Design review of the part built by this model. Coordinates are the model's own, in mm. A direction names the side the tool comes from. Round coordinates to 2 decimals unless told otherwise and drop trailing zeros. Order: outer loops, then holes, each group sorted by start corner. A loop starts at its lowest first (then second) coordinate and runs counter-clockwise, first axis right, second up. Notation, with made-up numbers: (88.25, -26.5) - (136.25, -26.5) arc R32 cw to (136.25, 8.5) - close; hole circle Ø5 at (23, 71). An arc over 180 degrees is marked (long way). Write item = value, one per line.
from build123d import *

# Parameters (mm, degrees)
CYLINDER2172_R               = 56
CYLINDER2172_DEPTH           = 7
CYLINDER2171_R               = 51
CYLINDER2171_DEPTH           = 7
BOX1045_W                    = 1.4
BOX1045_H                    = 60
BOX1045_DEPTH                = 7
BOX1045_PLACEMENT_ANGLE      = 19.7
BOX1044_W                    = 1.4
BOX1044_H                    = 60
BOX1044_DEPTH                = 7
BOX1044_PLACEMENT_ANGLE      = 18
CUT727_PLACEMENT_ANGLE       = 45
BOX1038_W                    = 60
BOX1038_H                    = 60
BOX1038_DEPTH                = 7
BOX1038_PLACEMENT_ANGLE      = 1
BOX1036_W                    = 60
BOX1036_H                    = 60
BOX1036_DEPTH                = 7
BOX1036_PLACEMENT_ANGLE      = 2
BOX1043_W                    = 120
BOX1043_H                    = 60
BOX1043_DEPTH                = 7
TUBE090_R                    = 54.4
TUBE090_R_2                  = 53
TUBE090_DEPTH                = 7
BOX1041_W                    = 60
BOX1041_H                    = 60
BOX1041_DEPTH                = 7
BOX1041_PLACEMENT_ANGLE      = 20
BOX1039_W                    = 60
BOX1039_H                    = 60
BOX1039_DEPTH                = 7
BOX1039_PLACEMENT_ANGLE      = 20
BOX1037_W                    = 120
BOX1037_H                    = 60
BOX1037_DEPTH                = 7
TUBE091_R                    = 53.4
TUBE091_R_2                  = 52
TUBE091_DEPTH                = 7
CUT721_PLACEMENT_ANGLE       = 45
CYLINDER2170_R               = 51
CYLINDER2170_DEPTH           = 7
BOX1042_W                    = 1.4
BOX1042_H                    = 60
BOX1042_DEPTH                = 7
BOX1042_PLACEMENT_ANGLE      = 2.7
BOX1040_W                    = 1.4
BOX1040_H                    = 60
BOX1040_DEPTH                = 7
BOX1040_PLACEMENT_ANGLE      = 2
CUT722_PLACEMENT_ANGLE       = 45
CYLINDER2129_R               = 1.5
CYLINDER2129_DEPTH           = 100
CYLINDER2130_R               = 1.5
CYLINDER2130_DEPTH           = 100
CYLINDER2130_PLACEMENT_ANGLE = 145
CYLINDER2131_R               = 1.5
CYLINDER2131_DEPTH           = 100
CYLINDER2132_R               = 1.5
CYLINDER2132_DEPTH           = 100
CYLINDER2132_PLACEMENT_ANGLE = 225
CYLINDER2133_R               = 1.5
CYLINDER2133_DEPTH           = 100
CYLINDER2134_R               = 1.5
CYLINDER2134_DEPTH           = 100
CYLINDER2134_PLACEMENT_ANGLE = 45
CYLINDER2127_R               = 1.5
CYLINDER2127_DEPTH           = 100
CYLINDER2128_R               = 1.5
CYLINDER2128_DEPTH           = 100
CYLINDER2128_PLACEMENT_ANGLE = 45
TUBE092_R                    = 57
TUBE092_R_2                  = 32
TUBE092_DEPTH                = 10


with BuildPart() as obj1:
    # Cylinder2172 → Cylinder2172 (new body)
    with BuildSketch(Plane.XY.offset(45)):
        Circle(CYLINDER2172_R)
    extrude(amount=CYLINDER2172_DEPTH)


with BuildPart() as obj2:
    # Cylinder2171 → Cylinder2171 (new body)
    with BuildSketch(Plane.XY.offset(-22)):
        Circle(CYLINDER2171_R)
    extrude(amount=CYLINDER2171_DEPTH)


with BuildPart() as krychle1045:
    # Box1045 → Box1045 (new body)
    with BuildSketch(Plane.XY):
        with Locations((0.7, 30)):
            Rectangle(BOX1045_W, BOX1045_H)
    extrude(amount=BOX1045_DEPTH)


with BuildPart() as krychle1045_1:
    # Box1045 placement: moved
    add(krychle1045.part.moved(Location((0, 0, -22))).rotate(Axis((0, 0, -22), (0, 0, 1)), BOX1045_PLACEMENT_ANGLE))


with BuildPart() as common:
    # Box1044 → Box1044 (new body)
    with BuildSketch(Plane.XY):
        with Locations((0.7, 30)):
            Rectangle(BOX1044_W, BOX1044_H)
    extrude(amount=BOX1044_DEPTH)


with BuildPart() as common_1:
    # Box1044 placement: moved
    add(common.part.moved(Location((0, 0, -22))).rotate(Axis((0, 0, -22), (0, 0, -1)), BOX1044_PLACEMENT_ANGLE))

    # Compound1133: union Krychle1045
    add(krychle1045_1.part)

    # Cut727: cut obj2
    add(obj2.part, mode=Mode.SUBTRACT)


with BuildPart() as common_2:
    # Cut727 placement: moved
    add(common_1.part.moved(Location((0, 0, 67))).rotate(Axis((0, 0, 67), (0, 0, 1)), CUT727_PLACEMENT_ANGLE))

    # Common: intersect obj1
    add(obj1.part, mode=Mode.INTERSECT)


with BuildPart() as krychle1038:
    # Box1038 → Box1038 (new body)
    with BuildSketch(Plane.XY):
        with Locations((30, 30)):
            Rectangle(BOX1038_W, BOX1038_H)
    extrude(amount=BOX1038_DEPTH)


with BuildPart() as krychle1038_1:
    # Box1038 placement: moved
    add(krychle1038.part.moved(Location((-59.990862, -1.047144, -22))).rotate(Axis((-59.990862, -1.047144, -22), (0, 0, 1)), BOX1038_PLACEMENT_ANGLE))


with BuildPart() as compound1130:
    # Box1036 → Box1036 (new body)
    with BuildSketch(Plane.XY):
        with Locations((30, 30)):
            Rectangle(BOX1036_W, BOX1036_H)
    extrude(amount=BOX1036_DEPTH)


with BuildPart() as compound1130_1:
    # Box1036 placement: moved
    add(compound1130.part.moved(Location((0, 0, -22))).rotate(Axis((0, 0, -22), (0, 0, -1)), BOX1036_PLACEMENT_ANGLE))

    # Compound1130: union Krychle1038
    add(krychle1038_1.part)


with BuildPart() as krychle1043:
    # Box1043 → Box1043 (new body)
    with BuildSketch(Plane(origin=(-60, -60, -22), x_dir=(1, 0, 0), z_dir=(0, 0, 1))):
        with Locations((60, 30)):
            Rectangle(BOX1043_W, BOX1043_H)
    extrude(amount=BOX1043_DEPTH)


with BuildPart() as cut723:
    # Tube090 → Tube090 (new body)
    with BuildSketch(Plane.XY.offset(-22)):
        Circle(TUBE090_R)
        Circle(TUBE090_R_2, mode=Mode.SUBTRACT)
    extrude(amount=TUBE090_DEPTH)

    # Cut726: cut Krychle1043
    add(krychle1043.part, mode=Mode.SUBTRACT)

    # Cut723: cut Compound1130
    add(compound1130_1.part, mode=Mode.SUBTRACT)


with BuildPart() as cut723_1:
    # Cut723 placement: moved
    add(cut723.part.moved(Location((0, 0, -7))))


with BuildPart() as krychle1041:
    # Box1041 → Box1041 (new body)
    with BuildSketch(Plane.XY):
        with Locations((30, 30)):
            Rectangle(BOX1041_W, BOX1041_H)
    extrude(amount=BOX1041_DEPTH)


with BuildPart() as krychle1041_1:
    # Box1041 placement: moved
    add(krychle1041.part.moved(Location((-56.381557, -20.521209, -22))).rotate(Axis((-56.381557, -20.521209, -22), (0, 0, 1)), BOX1041_PLACEMENT_ANGLE))


with BuildPart() as compound1129:
    # Box1039 → Box1039 (new body)
    with BuildSketch(Plane.XY):
        with Locations((30, 30)):
            Rectangle(BOX1039_W, BOX1039_H)
    extrude(amount=BOX1039_DEPTH)


with BuildPart() as compound1129_1:
    # Box1039 placement: moved
    add(compound1129.part.moved(Location((0, 0, -22))).rotate(Axis((0, 0, -22), (0, 0, -1)), BOX1039_PLACEMENT_ANGLE))

    # Compound1129: union Krychle1041
    add(krychle1041_1.part)


with BuildPart() as krychle1037:
    # Box1037 → Box1037 (new body)
    with BuildSketch(Plane(origin=(-60, -60, -22), x_dir=(1, 0, 0), z_dir=(0, 0, 1))):
        with Locations((60, 30)):
            Rectangle(BOX1037_W, BOX1037_H)
    extrude(amount=BOX1037_DEPTH)


with BuildPart() as cut721:
    # Tube091 → Tube091 (new body)
    with BuildSketch(Plane.XY.offset(-22)):
        Circle(TUBE091_R)
        Circle(TUBE091_R_2, mode=Mode.SUBTRACT)
    extrude(amount=TUBE091_DEPTH)

    # Cut718: cut Krychle1037
    add(krychle1037.part, mode=Mode.SUBTRACT)

    # Cut724: cut Compound1129
    add(compound1129_1.part, mode=Mode.SUBTRACT)


with BuildPart() as cut721_1:
    # Cut724 placement: moved
    add(cut721.part.moved(Location((0, 0, -7))))

    # Cut721: cut Cut723
    add(cut723_1.part, mode=Mode.SUBTRACT)


with BuildPart() as cut721_2:
    # Cut721 placement: moved
    add(cut721_1.part.moved(Location((0, 0, 74))).rotate(Axis((0, 0, 74), (0, 0, 1)), CUT721_PLACEMENT_ANGLE))


with BuildPart() as obj3:
    # Cylinder2170 → Cylinder2170 (new body)
    with BuildSketch(Plane.XY.offset(-22)):
        Circle(CYLINDER2170_R)
    extrude(amount=CYLINDER2170_DEPTH)


with BuildPart() as krychle1042:
    # Box1042 → Box1042 (new body)
    with BuildSketch(Plane.XY):
        with Locations((0.7, 30)):
            Rectangle(BOX1042_W, BOX1042_H)
    extrude(amount=BOX1042_DEPTH)


with BuildPart() as krychle1042_1:
    # Box1042 placement: moved
    add(krychle1042.part.moved(Location((0, 0, -22))).rotate(Axis((0, 0, -22), (0, 0, 1)), BOX1042_PLACEMENT_ANGLE))


with BuildPart() as cut722:
    # Box1040 → Box1040 (new body)
    with BuildSketch(Plane.XY):
        with Locations((0.7, 30)):
            Rectangle(BOX1040_W, BOX1040_H)
    extrude(amount=BOX1040_DEPTH)


with BuildPart() as cut722_1:
    # Box1040 placement: moved
    add(cut722.part.moved(Location((0, 0, -22))).rotate(Axis((0, 0, -22), (0, 0, -1)), BOX1040_PLACEMENT_ANGLE))

    # Compound1131: union Krychle1042
    add(krychle1042_1.part)

    # Cut722: cut obj3
    add(obj3.part, mode=Mode.SUBTRACT)


with BuildPart() as cut722_2:
    # Cut722 placement: moved
    add(cut722_1.part.moved(Location((0, 0, 67))).rotate(Axis((0, 0, 67), (0, 0, 1)), CUT722_PLACEMENT_ANGLE))


with BuildPart() as obj4:
    # Cylinder2129 → Cylinder2129 (new body)
    with BuildSketch(Plane(origin=(38, 0, 0), x_dir=(0, 1, 0), z_dir=(0, 0, 1))):
        Circle(CYLINDER2129_R)
    extrude(amount=CYLINDER2129_DEPTH)


with BuildPart() as obj5:
    # Cylinder2130 → Cylinder2130 (new body)
    with BuildSketch(Plane.XY):
        Circle(CYLINDER2130_R)
    extrude(amount=CYLINDER2130_DEPTH)


with BuildPart() as obj5_1:
    # Cylinder2130 placement: moved
    add(obj5.part.moved(Location((21.795905, 31.127778, 0))).rotate(Axis((21.795905, 31.127778, 0), (0, 0, 1)), CYLINDER2130_PLACEMENT_ANGLE))


with BuildPart() as obj6:
    # Cylinder2131 → Cylinder2131 (new body)
    with BuildSketch(Plane(origin=(0, 38, 0), x_dir=(-1, 0, 0), z_dir=(0, 0, 1))):
        Circle(CYLINDER2131_R)
    extrude(amount=CYLINDER2131_DEPTH)


with BuildPart() as obj7:
    # Cylinder2132 → Cylinder2132 (new body)
    with BuildSketch(Plane.XY):
        Circle(CYLINDER2132_R)
    extrude(amount=CYLINDER2132_DEPTH)


with BuildPart() as obj7_1:
    # Cylinder2132 placement: moved
    add(obj7.part.moved(Location((-26.870058, 26.870058, 0))).rotate(Axis((-26.870058, 26.870058, 0), (0, 0, 1)), CYLINDER2132_PLACEMENT_ANGLE))


with BuildPart() as obj8:
    # Cylinder2133 → Cylinder2133 (new body)
    with BuildSketch(Plane(origin=(-38, 0, 0), x_dir=(0, -1, 0), z_dir=(0, 0, 1))):
        Circle(CYLINDER2133_R)
    extrude(amount=CYLINDER2133_DEPTH)


with BuildPart() as obj9:
    # Cylinder2134 → Cylinder2134 (new body)
    with BuildSketch(Plane.XY):
        Circle(CYLINDER2134_R)
    extrude(amount=CYLINDER2134_DEPTH)


with BuildPart() as obj9_1:
    # Cylinder2134 placement: moved
    add(obj9.part.moved(Location((-26.870058, -26.870058, 0))).rotate(Axis((-26.870058, -26.870058, 0), (0, 0, -1)), CYLINDER2134_PLACEMENT_ANGLE))


with BuildPart() as obj10:
    # Cylinder2127 → Cylinder2127 (new body)
    with BuildSketch(Plane(origin=(0, -38, 0), x_dir=(1, 0, 0), z_dir=(0, 0, 1))):
        Circle(CYLINDER2127_R)
    extrude(amount=CYLINDER2127_DEPTH)


with BuildPart() as compound1132:
    # Cylinder2128 → Cylinder2128 (new body)
    with BuildSketch(Plane.XY):
        Circle(CYLINDER2128_R)
    extrude(amount=CYLINDER2128_DEPTH)


with BuildPart() as compound1132_1:
    # Cylinder2128 placement: moved
    add(compound1132.part.moved(Location((26.870058, -26.870058, 0))).rotate(Axis((26.870058, -26.870058, 0), (0, 0, 1)), CYLINDER2128_PLACEMENT_ANGLE))

    # Compound1132: union obj4, obj5, obj6, obj7, obj8, obj9, obj10
    add(obj4.part)
    add(obj5_1.part)
    add(obj6.part)
    add(obj7_1.part)
    add(obj8.part)
    add(obj9_1.part)
    add(obj10.part)


with BuildPart() as cut728:
    # Tube092 → Tube092 (new body)
    with BuildSketch(Plane.XY.offset(42)):
        Circle(TUBE092_R)
        Circle(TUBE092_R_2, mode=Mode.SUBTRACT)
    extrude(amount=TUBE092_DEPTH)

    # Cut725: cut Compound1132
    add(compound1132_1.part, mode=Mode.SUBTRACT)

    # Cut719: cut Cut722
    add(cut722_2.part, mode=Mode.SUBTRACT)

    # Cut720: cut Cut721
    add(cut721_2.part, mode=Mode.SUBTRACT)

    # Cut728: cut Common
    add(common_2.part, mode=Mode.SUBTRACT)


solid = cut728.part
Item 1: Take a section at A-A, the plane x = 0. State the section outline as (y, z) points, and give its area (3 significant figures).
Data:
outline = (-57, 42) - (-39.5, 42) - (-39.5, 52) - (-57, 52) - close; (-36.5, 42) - (-32, 42) - (-32, 52) - (-36.5, 52) - close; (32, 42) - (36.5, 42) - (36.5, 52) - (32, 52) - close; (39.5, 42) - (57, 42) - (57, 52) - (39.5, 52) - close
area = 440 mm2
Item 2: Take a section at D-D, the plane z = 48. Count the separate pieces of the cut face and the enclosed holes in it, and give its area (3 significant figures).
Data:
separate_pieces = 2
enclosed_holes = 9
area = 6,860 mm2
Item 3: Insertion check: P1, Ø6, axis at x = 31, z = 49.5, coming from the -Y side. The pin has a flat end and moves straight along its axis. Give the tip position at first contact, or say it passes through.
Data:
P1 = -49.65
Item 4: For faces 4 (the face through (-39.9, 38.2, 48.5)), 5 (the face through (39.464, -0.325, 46.93)), list the 3-axis set-ups (+Z, -Z, +X, -X, +Y, -Y) from which the entire face can be reached by the end or side of a thin tool; tool diameter is ignored.
Data:
face_4 = +Z
face_5 = +Z, -Z
Item 5: The part is to be moulded in two halves that separate along Y. For faces 1 (the face through (25, -25, 52)), 2 (the face through (-0.325, -39.464, 46.93)), 3 (the face through (26.3, -50.57, 46.93)), say which applies: +Y half, -Y half, draft (parallel to the pull), parting line (faces both ways), or undercut.
Data:
face_1 = draft
face_2 = undercut
face_3 = parting line
Item 6: For line 1 along Y through (x, z) = (0, 48.5); line 2 along X through (y, z) = (26, 51); line 3 along Y through (x, z) = (22, 51), list the stretches that pass through material, from the lowest coordinate up. Write a range as [from, to].
Data:
line_1 = [-57, -39.5], [-36.5, -32], [32, 36.5], [39.5, 57]
line_2 = [-50.72, -46.64], [-45.03, -28.09], [-25.65, -18.65], [18.65, 50.72]
line_3 = [-52.58, -23.24], [23.24, 29.64], [32.61, 52.58]
Item 7: Take a section at B-B, the plane y = -38. State the section outline as (x, z) points, and give its area (3 significant figures).
Data:
outline = (-42.49, 42) - (-1.5, 42) - (-1.5, 52) - (-42.49, 52) - close; (1.5, 42) - (42.49, 42) - (42.49, 52) - (1.5, 52) - close
area = 820 mm2
